Design review of the part built by this model. Coordinates are the model's own, in mm. Face numbers are marked on the shaded views. A direction names the side the tool comes from. Give positions to 0.01 mm unless a question says otherwise; leave off trailing zeros. Write each loop counter-clockwise with the first axis right and the second up, starting at its lowest first coordinate (ties: lowest second). Pieces come first, ordered by that corner, then holes. Notation, with made-up numbers: (3.25, 79.5) - (50.25, 79.5) arc R23 ccw to (50.25, 91.5) - close; hole circle Ø10 at (4.5, -38.75). An arc over 180 degrees is marked (long way). Write each question's results on one line, items separated by ' | '. Start each with the question number.
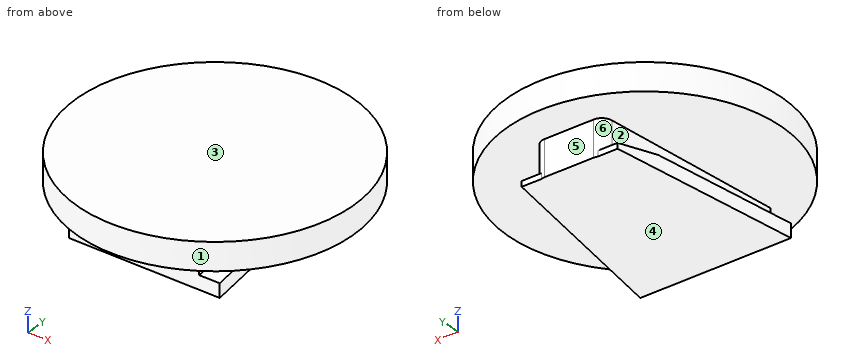
from build123d import *

# Parameters (mm, degrees)
F1_DEPTH      = 1.5875
F3_DEPTH      = 17.4635
F5_DEPTH      = 2.54
F5_DEPTH_BACK = 1.5875
F6_R          = 15.875
F7_DEPTH      = 3.175


with BuildPart() as f1:
    # F0 (on Top) → F1 (new body)
    with BuildSketch(Plane.XY):
        Polygon((3.175, 22.225), (0, 0), (17.4625, 0), (14.2875, 22.225), (8.73125, 22.225), align=None)
    extrude(amount=F1_DEPTH)

    # F2 (on Right) → F3 (cut, through all)
    with BuildSketch(Plane.YZ):
        Polygon((5.840029, 3.627038), (22.225, 0.635), (22.723673, 7.972618), (5.840029, 7.972618), align=None)
    extrude(amount=F3_DEPTH, mode=Mode.SUBTRACT)

    # F4 (on face) → F5 (join, two sides)
    with BuildSketch(Plane.XY.offset(1.5875)) as f5_sk:
        with BuildLine():
            Line((2.38125, 0), (8.73125, 0))
            Line((8.73125, 0), (15.08125, 0))
            Line((15.08125, 0), (12.821199, 21.168127))
            ThreePointArc((12.821199, 21.168127), (12.407396, 21.977792), (11.558376, 22.3033))
            Line((11.558376, 22.3033), (8.73125, 22.3033))
            Line((8.73125, 22.3033), (5.904124, 22.3033))
            ThreePointArc((5.904124, 22.3033), (5.055104, 21.977792), (4.641301, 21.168127))
            Line((4.641301, 21.168127), (2.38125, 0))
        make_face()
    extrude(amount=F5_DEPTH)
    extrude(f5_sk.sketch, amount=-F5_DEPTH_BACK)

    # F6 (on face) → F7 (join)
    with BuildSketch(Plane.XY.offset(4.1275)):
        with Locations((8.73125, 10.752532)):
            Circle(F6_R)
    extrude(amount=F7_DEPTH)


solid = f1.part
Q1. Add section A-A on y = 10. State the section outline as (x, z) points.
Q2. Add section D-D on y = 15.5. State the section outline as (x, z) points, plus the area to 3 significant figures.
Q3. Add section B-B on z = 3.25. State the section outline as (x, y) points.
Q4. For line 1 along Z through (x, y) = (22.5, 7); line 2 along X through (y, z) = (2, 6.5); line 3 along X through (y, z) = (6, 3), list the stretches that pass through material, from the lowest coordinate up. Write a range as [from, to].
Q5. Insertion check: P1, Ø1.2, axis at x = 7.5, z = 2.5, coming from the -Y side; P2, Ø0.5, axis at x = 4.5, z = 0.5, coming from the +Y side (3 decimals). Each pin has a flat end and moves straight along its axis. Give the tip position at first contact, or say it passes through.
Q6. Machinability: for the marked faces 5 and 6, which of the approach directions +Z, -Z, +X, -X, +Y, -Y give a long, thin tool a straight path to every point of the face, cutting with its end or side? Answer none if there is none.
Q7. Add section C-C on x = 7.5. State the section outline as (y, z) points, plus the area to 3 significant figures.
Q8. The part is to be moulded in two halves that separate along Z. For the marked faces 1, 2, 3 and 4, say which applies: +Z half, -Z half, draft (parallel to the pull), parting line (faces both ways), or undercut.
Result:
1) outline: (-7.13, 4.13) - (3.45, 4.13) - (3.45, 1.59) - (1.43, 1.59) - (1.43, 0) - (16.03, 0) - (16.03, 1.59) - (14.01, 1.59) - (14.01, 4.13) - (24.59, 4.13) - (24.59, 7.3) - (-7.13, 7.3) - close
2) outline: (-6.42, 4.13) - (4.04, 4.13) - (4.04, 1.59) - (2.21, 1.59) - (2.21, 0) - (15.25, 0) - (15.25, 1.59) - (13.43, 1.59) - (13.43, 4.13) - (23.88, 4.13) - (23.88, 7.3) - (-6.42, 7.3) - close | area: 141 mm²
3) outline: (2.38, 0) - (15.08, 0) - (12.82, 21.17) arc R1.27 ccw to (11.56, 22.3) - (5.9, 22.3) arc R1.27 ccw to (4.64, 21.17) - close
4) line 1: z = [4.13, 7.3] | line 2: x = [-4.51, 21.98] | line 3: x = [3.02, 14.44]
5) P1: stops at y = 0 | P2: stops at y = 22.225
6) face 5: -Z, +X, -X, +Y | face 6: -X, +Y
7) outline: (-5.07, 4.13) - (0, 4.13) - (0, 0) - (22.3, 0) - (22.3, 4.13) - (26.58, 4.13) - (26.58, 7.3) - (-5.07, 7.3) - close | area: 193 mm²
8) face 1: draft | face 2: undercut | face 3: +Z half | face 4: -Z half
